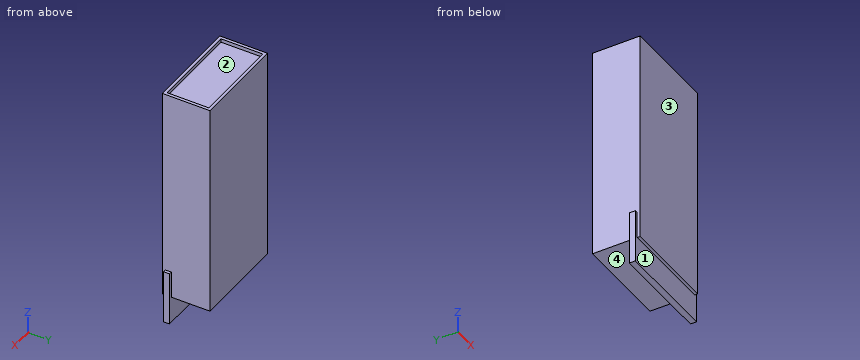
```python
from build123d import *

# Parameters (mm, degrees)
SKETCH_1_W          = 800
SKETCH_1_H          = 400
EXTRUDE_1_DEPTH     = 1800
SKETCH_2_W          = 750
SKETCH_2_H          = 350
CUT_EXTRUDE_1_DEPTH = 30
SKETCH_3_W          = 750
SKETCH_3_H          = 20
EXTRUDE_2_DEPTH     = 800
SKETCH_4_R          = 20
EXTRUDE_3_DEPTH     = 50
SKETCH_5_W          = 850
SKETCH_5_H          = 450
EXTRUDE_4_DEPTH     = 50


with BuildPart() as part:
    # 草图1 → 凸台-拉伸1 (new body)
    with BuildSketch(Plane.XY):
        Rectangle(SKETCH_1_W, SKETCH_1_H)
    extrude(amount=EXTRUDE_1_DEPTH)

    # 草图2 → 切除-拉伸1 (cut)
    with BuildSketch(Plane.XY.offset(1800)):
        Rectangle(SKETCH_2_W, SKETCH_2_H)
    extrude(amount=-CUT_EXTRUDE_1_DEPTH, mode=Mode.SUBTRACT)

    # 草图3 → 凸台-拉伸2 (add)
    with BuildSketch(Plane.XY):
        with Locations((0, -180)):
            Rectangle(SKETCH_3_W, SKETCH_3_H)
    extrude(amount=EXTRUDE_2_DEPTH)

    # 草图4 → 凸台-拉伸3 (add)
    with BuildSketch(Plane.XY):
        with Locations((300, -180)):
            Circle(SKETCH_4_R)
    extrude(amount=EXTRUDE_3_DEPTH)

    # 草图5 → 凸台-拉伸4 (add)
    with BuildSketch(Plane(origin=(0, -175, 0), x_dir=(1, 0, 0), z_dir=(0, 1, 0))):
        Rectangle(SKETCH_5_W, SKETCH_5_H)
    extrude(amount=EXTRUDE_4_DEPTH)


solid = part.part
```
CAD build for the part. Positions are in the model's coordinates, mm. Face numbers are marked on the shaded views. A direction names the side the tool comes from. Coordinates: 2 decimals unless noted, no trailing zeros. Order: outer loops, then holes, each group sorted by start corner. A loop starts at its lowest first (then second) coordinate and runs counter-clockwise, first axis right, second up. Notation, with made-up numbers: M 39.25,-13 L 56.25,-13 A19 ccw 56.25,3 Z; hole C 88,86 d10. An arc over 180 degrees is marked long. Write each question's results on one line, items separated by ' | '. Start each with the question number.
Q1. Flat gauge pins, fed straight in: P1, Ø6, axis at x = -286.5, y = 92.5, coming from the +Z side; P2, Ø20, axis at x = -418.5, y = -138.5, coming from the +Z side; P3, Ø1.5, axis at y = 160, z = 404.5, coming from the -X side. Where does each tip first touch, or does it go through?
Q2. Which spindle directions (+Z, -Z, +X, -X, +Y, -Y) get a long thin tool onto all of the face, cutting with end or side? Do the marked faces 3 and 4. Say none if no direction does.
Q3. Pull direction X, two halves, no side cores. Call the marked faces 1 and 2: +X half, -X half, draft (parallel to the pull), parting line (faces both ways), or undercut.
Q4. Drill centre lines: probe 1 along Z at (x, y) = (184.5, 97.5); probe 2 along X at (y, z) = (0, 90.5); probe 3 along Z at (x, y) = (274.5, 182). Where is each one in solid material? Low to high. Write a range as from..to.
Q5. Cut at A-A (y = 139.5). List the corners of the cut face in (x, z).
Q6. Cut at C-C (z = 1303.5). List the corners of the cut face in (x, y), then the cut area to 3 significant figures.
Q7. Cut at B-B (x = -182). List the corners of the cut face in (y, z), then the cut area to 3 significant figures.
Found:
1) P1: z = 1770 | P2: z = 225 | P3: x = -400
2) face 3: +Z, -Z, +X, -X, -Y | face 4: -Z, +X, -X, +Y
3) face 1: draft | face 2: undercut
4) probe 1: 0..1770 | probe 2: -400..400 | probe 3: 0..1800
5) outline: M -400,0 L 400,0 L 400,1800 L 375,1800 L 375,1770 L -375,1770 L -375,1800 L -400,1800 Z
6) outline: M -400,-200 L 400,-200 L 400,200 L -400,200 Z | area: 320,000 mm²
7) outline: M -200,0 L -175,0 L -175,-225 L -125,-225 L -125,0 L 200,0 L 200,1800 L 175,1800 L 175,1770 L -175,1770 L -175,1800 L -200,1800 Z | area: 721,000 mm²
